```python
from build123d import *

# Parameters (mm, degrees)
BOSS_EXTRUDE1_DEPTH                       = 1.016
CSK_FOR_6_FLAT_HEAD_MACHINE_SCREW_2_COUNT = 2
CSK_FOR_6_FLAT_HEAD_MACHINE_SCREW_2_PITCH = 95.461432003
CSK_FOR_6_FLAT_HEAD_MACHINE_SCREW_3_COUNT = 2
CSK_FOR_6_FLAT_HEAD_MACHINE_SCREW_3_PITCH = 121.190211651
CSK_FOR_6_FLAT_HEAD_MACHINE_SCREW_4_COUNT = 2
CSK_FOR_6_FLAT_HEAD_MACHINE_SCREW_4_PITCH = 81.28
M3_CLEARANCE_HOLE1_D                      = 3.4
M3_CLEARANCE_HOLE1_DEPTH                  = 20.066
M3_CLEARANCE_HOLE1_TIP                    = 1.021463052


with BuildPart() as part:
    # Sketch1 → Boss-Extrude1 (new body)
    with BuildSketch(Plane(origin=(0, 0, 0), x_dir=(1, 0, 0), z_dir=(0, 1, 0))):
        Polygon((-107.95, 50.8), (-131.7625, 50.8), (-131.7625, 107.95), (-107.95, 107.95), (-107.95, 158.75), (0, 158.75), (0, 107.95), (23.876, 107.95), (23.876, 50.8), (0, 50.8), (0, 0), (-107.95, 0), align=None)
    extrude(amount=BOSS_EXTRUDE1_DEPTH)

    # Sketch2 → CSK for #6 Flat Head Machine Screw (100)1 (revolve, cut)
    with BuildSketch(Plane(origin=(-101.6, 1.016, -116.84), x_dir=(0, 0, 1), z_dir=(1, 0, 0))):
        Polygon((0, 0), (0, 1.016), (1.89865, 1.016), (1.89865, 1.380025208), (3.5433, 0), align=None)
    csk_for_6_flat_head_machine_screw_100 = revolve(axis=Axis((-101.6, 7.366, -116.84), (0, -1, 0)), mode=Mode.SUBTRACT)

    # CSK for _6 Flat Head Machine Screw _ 2: CSK for #6 Flat Head Machine Screw (100)1 ×2
    with Locations(*[Vector(0.997785157856609, 0, -0.06651901052377401) * (i * CSK_FOR_6_FLAT_HEAD_MACHINE_SCREW_2_PITCH) for i in range(1, CSK_FOR_6_FLAT_HEAD_MACHINE_SCREW_2_COUNT)]):
        add(csk_for_6_flat_head_machine_screw_100, mode=Mode.SUBTRACT)

    # CSK for _6 Flat Head Machine Screw _ 3: CSK for #6 Flat Head Machine Screw (100)1 ×2
    with Locations(*[Vector(0.7859545643367972, 0, 0.6182842572782808) * (i * CSK_FOR_6_FLAT_HEAD_MACHINE_SCREW_3_PITCH) for i in range(1, CSK_FOR_6_FLAT_HEAD_MACHINE_SCREW_3_COUNT)]):
        add(csk_for_6_flat_head_machine_screw_100, mode=Mode.SUBTRACT)

    # CSK for _6 Flat Head Machine Screw _ 4: CSK for #6 Flat Head Machine Screw (100)1 ×2
    with Locations(*[(0, 0, i * CSK_FOR_6_FLAT_HEAD_MACHINE_SCREW_4_PITCH) for i in range(1, CSK_FOR_6_FLAT_HEAD_MACHINE_SCREW_4_COUNT)]):
        add(csk_for_6_flat_head_machine_screw_100, mode=Mode.SUBTRACT)

    # M3 Clearance Hole1
    with Locations(Plane(origin=(0, 1.016, 0), x_dir=(1, 0, 0), z_dir=(0, 1, 0))):
        with Locations((-63.846986831, 94.548500407), (-63.621171585, 82.731605313), (-75.641328415, 95.312377887), (-75.415513169, 83.495482793)):
            Hole(M3_CLEARANCE_HOLE1_D / 2, depth=M3_CLEARANCE_HOLE1_DEPTH)
            with Locations((0, 0, -(M3_CLEARANCE_HOLE1_DEPTH + M3_CLEARANCE_HOLE1_TIP / 2))):  # 118° drill point
                Cone(0, M3_CLEARANCE_HOLE1_D / 2, M3_CLEARANCE_HOLE1_TIP, mode=Mode.SUBTRACT)


solid = part.part
```
The model under review builds one solid part; all positions refer to its coordinate system, in mm. Round coordinates to 2 decimals unless told otherwise and drop trailing zeros. Order: outer loops, then holes, each group sorted by start corner. A loop starts at its lowest first (then second) coordinate and runs counter-clockwise, first axis right, second up. Notation, with made-up numbers: M -35.75,65 L 9.25,65 A27 cw 9.25,81 Z; hole C 43,-12 d6. An arc over 180 degrees is marked long. Use a Markdown table: item, result.
1) Consider section A-A (x = -6.35). Write out the cut boundary in (y, z).
Report:
| item | result |
|---|---|
| outline | M 0,-158.75 L 1.02,-158.75 L 1.02,-126.73 L 0,-125.52 Z; M 0,-120.86 L 1.02,-119.65 L 1.02,-45.45 L 0,-44.24 Z; M 0,-39.58 L 1.02,-38.37 L 1.02,0 L 0,0 Z |
2) Insertion check: pin 1 (4 mm diameter, centred on x = -44, z = -34.5, fed in from -Y); pin 2 (2.5 mm diameter, centred on x = -75.64, z = -95.31, fed in from -Y); pin 3 (0.5 mm diameter, centred on x = 16, y = 0.5, fed in from +Z); pin 4 (0.5 mm diameter, centred on x = 13, y = 0.5, fed in from -Z). Each pin has a flat end and moves straight along its axis. Give the tip position at first contact, or say it passes through.
Report:
| item | result |
|---|---|
| pin 1 | y = 0 |
| pin 2 | through |
| pin 3 | z = -50.8 |
| pin 4 | z = -107.95 |
3) Consider section C-C (z = -35.56). Write out the cut boundary in (x, y).
Report:
| item | result |
|---|---|
| outline | M -107.95,0 L -103.93,0 L -105.14,1.02 L -107.95,1.02 Z; M -99.27,0 L 0,0 L 0,1.02 L -98.06,1.02 Z |
4) Draft analysis for pull direction Z (two halves, no side actions). For faces 1 (the face through (-53, 1.016, -80)), 2 (the face through (-65.47, 0.5, -95.06)), state which applies: released by +Z, released by -Z, zero draft, split by the parting line, or undercut.
Report:
| item | result |
|---|---|
| face 1 | zero draft |
| face 2 | undercut |
5) Wall thickness on line 1 along X through (y, z) = (0.55, -96); line 2 along Z through (x, y) = (-102, 0.65); line 3 along Z through (x, y) = (-113, 0.2): over which ranges is each line inside the solid? List them lowest first. Write a range as [from, to].
Report:
| item | result |
|---|---|
| line 1 | [-131.76, -77.2], [-74.09, -64.73], [-62.96, 23.88] |
| line 2 | [-158.75, -119.92], [-113.76, -38.64], [-32.48, 0] |
| line 3 | [-107.95, -50.8] |
6) Consider section B-B (y = 0.2). Give the number of separate pieces and of enclosed holes in the cut face, then the cut area to 3 significant figures.
Report:
| item | result |
|---|---|
| separate pieces | 1 |
| enclosed holes | 8 |
| area | 19,700 mm^2 |
7) Consider section D-D (z = -111). Write out the cut boundary in (x, y), then the cut area to 3 significant figures.
Report:
| item | result |
|---|---|
| outline | M -107.95,0 L 0,0 L 0,1.02 L -107.95,1.02 Z |
| area | 110 mm^2 |
